Build history of the part. All positions in model axes, mm. A direction names the side the tool comes from. Round coordinates to 2 decimals unless told otherwise and drop trailing zeros. Order: outer loops, then holes, each group sorted by start corner. A loop starts at its lowest first (then second) coordinate and runs counter-clockwise, first axis right, second up. Notation, with made-up numbers: (32, -9) -> (89, -9) arc R16 ccw to (89, 18) -> close; hole circle Ø7 at (41.5, 54.25). An arc over 180 degrees is marked (long way). Write item = value, one per line.
from build123d import *

# Parameters (mm, degrees)
SKETCH1_W           = 115.0112
SKETCH1_H           = 70.993
BOSS_EXTRUDE1_DEPTH = 3.9878
SKETCH2_W           = 89.9922
SKETCH2_H           = 65.9892
BOSS_EXTRUDE2_DEPTH = 1.99898
BOSS_EXTRUDE3_DEPTH = 65.9892
CUT_EXTRUDE1_DEPTH  = 5.0038
SKETCH5_R           = 11.5062
BOSS_EXTRUDE4_DEPTH = 8.001
SKETCH6_R           = 0.99949
BOSS_EXTRUDE5_DEPTH = 10.0076


with BuildPart() as part:
    # Sketch1 → Boss-Extrude1 (new body)
    with BuildSketch(Plane(origin=(0, 0, 0), x_dir=(1, 0, 0), z_dir=(0, 1, 0))):
        with Locations((57.5056, 35.4965)):
            Rectangle(SKETCH1_W, SKETCH1_H)
    extrude(amount=BOSS_EXTRUDE1_DEPTH)

    # Sketch2 → Boss-Extrude2 (add)
    with BuildSketch(Plane(origin=(0, 3.9878, 0), x_dir=(1, 0, 0), z_dir=(0, 1, 0))):
        with Locations((62.5221, 35.9918)):
            Rectangle(SKETCH2_W, SKETCH2_H)
    extrude(amount=BOSS_EXTRUDE2_DEPTH)

    # Sketch3 → Boss-Extrude3 (add)
    with BuildSketch(Plane.XY.offset(-2.9972)):
        Polygon((17.526, 5.98678), (12.5222, 5.98678), (12.5222, 7.98576), (107.5182, 7.98576), (107.5182, 5.98678), align=None)
    extrude(amount=-BOSS_EXTRUDE3_DEPTH)

    # Sketch4 → Cut-Extrude1 (cut)
    with BuildSketch(Plane(origin=(0, 7.98576, 0), x_dir=(1, 0, 0), z_dir=(0, 1, 0))):
        with BuildLine():
            Line((33.5026, 14.986), (87.5284, 14.986))
            ThreePointArc((87.5284, 14.986), (88.228859977, 15.276140023), (88.519, 15.9766))
            Line((88.519, 15.9766), (88.519, 54.991))
            ThreePointArc((88.519, 54.991), (88.228859977, 55.691459977), (87.5284, 55.9816))
            Line((87.5284, 55.9816), (33.5026, 55.9816))
            ThreePointArc((33.5026, 55.9816), (32.802140023, 55.691459977), (32.512, 54.991))
            Line((32.512, 54.991), (32.512, 15.9766))
            ThreePointArc((32.512, 15.9766), (32.802140023, 15.276140023), (33.5026, 14.986))
        make_face()
    extrude(amount=-CUT_EXTRUDE1_DEPTH, mode=Mode.SUBTRACT)

    # Sketch5 → Boss-Extrude4 (add)
    with BuildSketch(Plane(origin=(0, 2.98196, 0), x_dir=(1, 0, 0), z_dir=(0, 1, 0))):
        with Locations((59.0042, 35.9918)):
            Circle(SKETCH5_R)
    extrude(amount=BOSS_EXTRUDE4_DEPTH)

    # Sketch6 → Boss-Extrude5 (add)
    with BuildSketch(Plane(origin=(115.0112, 0, 0), x_dir=(0, 0, -1), z_dir=(1, 0, 0))):
        with Locations((16.9926, 1.99898)):
            Circle(SKETCH6_R)
        with Locations((52.9844, 1.99898)):
            Circle(SKETCH6_R)
    extrude(amount=BOSS_EXTRUDE5_DEPTH)


solid = part.part
Q1. Cut at D-D, the plane x = 49.5. List the corners of the cut face in (y, z), and give its area (3 significant figures).
Check values:
outline = (0, -70.99) -> (3.99, -70.99) -> (3.99, -68.99) -> (7.99, -68.99) -> (7.99, -55.98) -> (2.98, -55.98) -> (2.98, -42.48) -> (10.98, -42.48) -> (10.98, -29.51) -> (2.98, -29.51) -> (2.98, -14.99) -> (7.99, -14.99) -> (7.99, -3) -> (3.99, -3) -> (3.99, 0) -> (0, 0) -> close
area = 446 mm²
Q2. Which spindle directions (+Z, -Z, +X, -X, +Y, -Y) get a long thin tool onto all of the face, cutting with end or side? Do faces 1 (the face through (59, 10.983, -36)), 2 (the face through (61, 6, -68.986)), 3 (the face through (61, 6, -55.982)), 4 (the face through (57, 2, -70.993)), 5 (the face through (61, 6, -2.997)). Say none if no direction does.
Check values:
face_1 = +Z, -Z, +X, -X, +Y
face_2 = -Z, +X, -X, +Y
face_3 = +Y
face_4 = -Z, +X, -X, +Y, -Y
face_5 = +Z, +X, -X, +Y
Q3. Flat gauge pins, fed straight in: pin 1 (2 mm diameter, centred on y = 6, z = -43.5, fed in from +X); pin 2 (1 mm diameter, centred on y = 7.5, z = -43.5, fed in from -X); pin 3 (3 mm diameter, centred on x = 88.5, y = 8, fed in from -Z). Where does each tip first touch, or does it go through?
Check values:
pin_1 = 107.52
pin_2 = 12.52
pin_3 = -68.99
Q4. Cut at B-B, the plane x = 31. List the corners of the cut face in (y, z), and give its area (3 significant figures).
Check values:
outline = (0, -70.99) -> (3.99, -70.99) -> (3.99, -68.99) -> (7.99, -68.99) -> (7.99, -3) -> (3.99, -3) -> (3.99, 0) -> (0, 0) -> close
area = 547 mm²
Q5. Cut at A-A, the plane z = -9. List the corners of the cut face in (x, y), and give its area (3 significant figures).
Check values:
outline = (0, 0) -> (115.01, 0) -> (115.01, 3.99) -> (107.52, 3.99) -> (107.52, 7.99) -> (12.52, 7.99) -> (12.52, 5.99) -> (17.53, 5.99) -> (17.53, 3.99) -> (0, 3.99) -> close
area = 828 mm²
Q6. Probe probe 1 along Y at (x, z) = (14.5, -43); probe 2 along Z at (x, y) = (46.5, 4.75); probe 3 along Y at (x, z) = (74.5, -47). List the from-to ranges inside material, lowest first.
Check values:
probe_1 = 0 to 3.99, 5.99 to 7.99
probe_2 = -68.99 to -55.98, -14.99 to -3
probe_3 = 0 to 2.98
Q7. Mould opens along X. For faces 6 (the face through (47.51, 6.93, -36.5)), 7 (the face through (107.518, 6, -36)), 8 (the face through (0, 2, -35)), 9 (the face through (15, 5.987, -36)) say: released by +X, released by -X, zero draft, split by the parting line, or undercut.
Check values:
face_6 = undercut
face_7 = released by +X
face_8 = released by -X
face_9 = zero draft
Q8. Cut at C-C, the plane z = -22. List the corners of the cut face in (x, y), and give its area (3 significant figures).
Check values:
outline = (0, 0) -> (115.01, 0) -> (115.01, 3.99) -> (107.52, 3.99) -> (107.52, 7.99) -> (88.52, 7.99) -> (88.52, 2.98) -> (32.51, 2.98) -> (32.51, 7.99) -> (12.52, 7.99) -> (12.52, 5.99) -> (17.53, 5.99) -> (17.53, 3.99) -> (0, 3.99) -> close
area = 548 mm²
